Here's how the part is built. I have some questions about the finished solid (model axes, mm). Face numbers are marked on the shaded views. A direction names the side the tool comes from. Round coordinates to 2 decimals unless told otherwise and drop trailing zeros. Order: outer loops, then holes, each group sorted by start corner. A loop starts at its lowest first (then second) coordinate and runs counter-clockwise, first axis right, second up. Notation, with made-up numbers: (11.5, 16.25) -> (27.5, 16.25) arc R32 cw to (27.5, 54.25) -> close; hole circle Ø2 at (76, -20). An arc over 180 degrees is marked (long way). Answer in a Markdown table with one row per item.
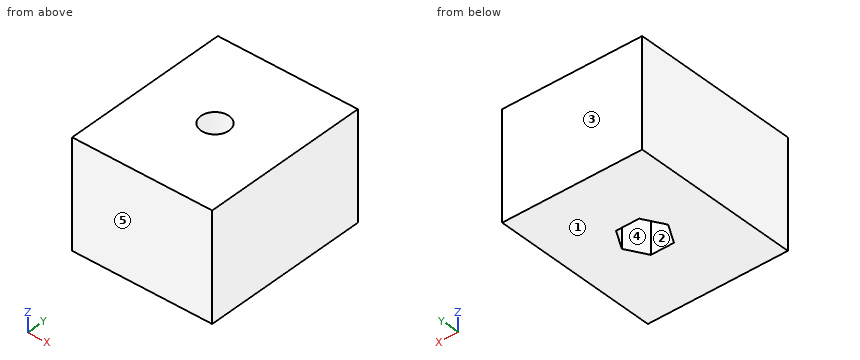
```python
from build123d import *

# Parameters (mm, degrees)
SKETCH1_W           = 16.9288177
SKETCH1_H           = 13
BOSS_EXTRUDE1_DEPTH = 10.16
SKETCH2_R           = 1.7
CUT_EXTRUDE1_DEPTH  = 9.906
SKETCH2_3_R         = 1.7
CUT_EXTRUDE2_DEPTH  = 15.748


with BuildPart() as part:
    # Sketch1 → Boss-Extrude1 (new, symmetric)
    with BuildSketch(Plane(origin=(0, 0, 0), x_dir=(1, 0, 0), z_dir=(0, 1, 0))):
        with Locations((0, 3.5)):
            Rectangle(SKETCH1_W, SKETCH1_H)
    extrude(amount=BOSS_EXTRUDE1_DEPTH, both=True)

    # Sketch2 → Cut-Extrude1 (cut)
    with BuildSketch(Plane(origin=(0, 0, -10), x_dir=(-1, 0, 0), z_dir=(0, 0, -1))):
        Polygon((-1.400074403, -2.425), (1.400074403, -2.425), (2.800148806, 0), (1.400074403, 2.425), (-1.400074403, 2.425), (-2.800148806, 0), align=None)
        Circle(SKETCH2_R, mode=Mode.SUBTRACT)
    extrude(amount=-CUT_EXTRUDE1_DEPTH, mode=Mode.SUBTRACT)

    # Sketch2_3 → Cut-Extrude2 (cut)
    with BuildSketch(Plane(origin=(0, 0, -10), x_dir=(-1, 0, 0), z_dir=(0, 0, -1))):
        Circle(SKETCH2_3_R)
    extrude(amount=-CUT_EXTRUDE2_DEPTH, mode=Mode.SUBTRACT)


solid = part.part
```
1. We'd pull the mould along Y, two halves only. Please class the marked faces 1, 2 and 3: released by +Y, released by -Y, zero draft, split by the parting line, or undercut.
Numbers:
| item | result |
|---|---|
| face 1 | zero draft |
| face 2 | undercut |
| face 3 | released by +Y |
2. Suppose I cut it at C-C on y = 1.25. Write out the boundary of the cut face in (x, z).
Numbers:
| item | result |
|---|---|
| outline | (-8.46, -10) -> (-2.08, -10) -> (-2.08, -0.09) -> (-1.15, -0.09) -> (-1.15, 3) -> (-8.46, 3) -> close; (1.15, -0.09) -> (2.08, -0.09) -> (2.08, -10) -> (8.46, -10) -> (8.46, 3) -> (1.15, 3) -> close |
3. Suppose I cut it at D-D on z = 0.75. Write out the boundary of the cut face in (x, y).
Numbers:
| item | result |
|---|---|
| outline | (-8.46, -10.16) -> (8.46, -10.16) -> (8.46, 10.16) -> (-8.46, 10.16) -> close; hole circle Ø3.4 at (0, 0) |
4. For pin 1 Ø1.5 at (x, y) = (-1, -0.5) entering from -Z, with a flat end and sliding along its axis, tell me the tip position at first contact or that it passes through.
Numbers:
| item | result |
|---|---|
| pin 1 | stops at z = -0.09 |
5. Please list where these lines run through material, in increasing order: line 1 along Y through (x, z) = (0, 1.55); line 2 along Y through (x, z) = (1.25, -2.5) (3 decimals).
Numbers:
| item | result |
|---|---|
| line 1 | y = -10.16 to -1.7, 1.7 to 10.16 |
| line 2 | y = -10.16 to -2.425, 2.425 to 10.16 |
6. Suppose I cut it at A-A on x = 0. Write out the boundary of the cut face in (y, z) (3 decimals), then the cut area to 3 significant figures.
Numbers:
| item | result |
|---|---|
| outline | (-10.16, -10) -> (-2.425, -10) -> (-2.425, -0.094) -> (-1.7, -0.094) -> (-1.7, 3) -> (-10.16, 3) -> close; (1.7, -0.094) -> (2.425, -0.094) -> (2.425, -10) -> (10.16, -10) -> (10.16, 3) -> (1.7, 3) -> close |
| area | 206 mm2 |
7. For the marked faces 4 and 5, which set-ups out of +Z, -Z, +X, -X, +Y, -Y let a thin tool reach every point of the face, with its end or its side?
Numbers:
| item | result |
|---|---|
| face 4 | -Z |
| face 5 | +Z, -Z, +X, -X, -Y |
8. Suppose I cut it at B-B on z = -4.25. Write out the boundary of the cut face in (x, y) (3 decimals), then the cut area to 3 significant figures.
Numbers:
| item | result |
|---|---|
| outline | (-8.464, -10.16) -> (8.464, -10.16) -> (8.464, 10.16) -> (-8.464, 10.16) -> close; hole (-2.8, 0) -> (-1.4, -2.425) -> (1.4, -2.425) -> (2.8, 0) -> (1.4, 2.425) -> (-1.4, 2.425) -> close |
| area | 324 mm2 |
